Work out the finished part from the listing and answer in its coordinate system (mm). A direction names the side the tool comes from. Coordinates: 2 decimals unless noted, no trailing zeros. Write each loop counter-clockwise with the first axis right and the second up, starting at its lowest first coordinate (ties: lowest second). Pieces come first, ordered by that corner, then holes. Notation, with made-up numbers: M -7.5,50.25 L 36.5,50.25 A15 ccw 36.5,66.25 Z; hole C 1,4.5 d4. An arc over 180 degrees is marked long. Use CSV: the item, a comma, the result in double quotes.
from build123d import *

# Parameters (mm, degrees)
F0_W     = 8
F0_H     = 4
F1_DEPTH = 10
F2_R     = 2.6
F3_DEPTH = 21
F4_R     = 2.6
F5_DEPTH = 50
F6_R     = 3


with BuildPart() as f1:
    # F0 (on Top) → F1 (new body)
    with BuildSketch(Plane.XY):
        with BuildLine():
            Line((20.489401, 8.474669), (20.489401, 14.474669))
            Line((20.489401, 14.474669), (5.543822, 14.474669))
            Line((5.543822, 14.474669), (5.543822, 34.474669))
            Line((5.543822, 34.474669), (-1.356178, 34.474669))
            Line((-1.356178, 34.474669), (-1.356178, 22.474669))
            Line((-1.356178, 22.474669), (-8.556178, 22.474669))
            Line((-8.556178, 22.474669), (-8.556178, 34.474669))
            Line((-8.556178, 34.474669), (-15.456178, 34.474669))
            Line((-15.456178, 34.474669), (-15.456178, 1.16472))
            ThreePointArc((-15.456178, 1.16472), (-11.149904, -10.767062), (0.624203, -15.487426))
            Line((0.624203, -15.487426), (11.585323, -15.487426))
            Line((11.585323, -15.487426), (20.489401, -15.487426))
            Line((20.489401, -15.487426), (20.489401, -7.487426))
            Line((20.489401, -7.487426), (8.728599, -7.487426))
            ThreePointArc((8.728599, -7.487426), (-11.479476, -0.686755), (7.773673, 8.474669))
            Line((7.773673, 8.474669), (20.489401, 8.474669))
        make_face()
        with Locations((13.989401, -11.487426)):
            Rectangle(F0_W, F0_H, mode=Mode.SUBTRACT)
    extrude(amount=F1_DEPTH)

    # F2 (on face) → F3 (cut, through all)
    with BuildSketch(Plane.YZ.offset(5.543822)):
        with BuildLine():
            ThreePointArc((34.474669, 5), (33.010203, 1.464466), (29.474669, 0))
            Line((29.474669, 0), (34.474669, 0))
            Line((34.474669, 0), (34.474669, 5))
        make_face()
        with BuildLine():
            ThreePointArc((29.474669, 10), (33.010203, 8.535534), (34.474669, 5))
            Line((34.474669, 5), (34.474669, 10))
            Line((34.474669, 10), (29.474669, 10))
        make_face()
        with Locations((29.474669, 5)):
            Circle(F2_R)
    extrude(amount=-F3_DEPTH, mode=Mode.SUBTRACT)

    # F4 (on face) → F5 (cut, symmetric)
    with BuildSketch(Plane(origin=(0, -13.487426, 0), x_dir=(-1, 0, 0), z_dir=(0, 1, 0))):
        with Locations((-13.989401, 5)):
            Circle(F4_R)
    extrude(amount=F5_DEPTH, both=True, mode=Mode.SUBTRACT)

    # F6
    f6_edges = [f1.edges().sort_by_distance(p)[0] for p in [
        (20.489401, 14.474669, 5),
        (20.489401, -7.487426, 5),
        (20.489401, -15.487426, 5),
    ]]
    fillet(f6_edges, radius=F6_R)


solid = f1.part
Item 1: A tool of negligible diameter and unlimited length cuts with its end or side. For faces 1 (the face through (-5, 22.475, 5)), 2 (the face through (5.544, 24, 5)), 3 (the face through (17.989, -12, 5)), 4 (the face through (15.5, 8.475, 2.7)), from which of +Z, -Z, +X, -X, +Y, -Y can it reach the whole face along a straight path? Write none if from no direction.
Answer:
face 1,"+Z, -Z, +Y"
face 2,"+Z, -Z, +X, +Y"
face 3,"+Z, -Z"
face 4,"+Z, -Z, +X"
Item 2: Consider probe 1 along Y at (x, z) = (16, 0.75); probe 2 along X at (y, z) = (28.5, 2); probe 3 along X at (y, z) = (10.5, 4.75). Determine where each line is inside the solid, lowest interval first.
Answer:
probe 1,"y = -15.49 to -13.49, -9.49 to -7.49, 8.47 to 14.47"
probe 2,"x = -15.46 to -8.56, -1.36 to 5.54"
probe 3,"x = -15.46 to -4.69, 4.69 to 11.4, 16.58 to 20.49"
Item 3: For a pull along Y with two mould halves and no side action, classify faces 5 (the face through (10, 14.475, 5)), 6 (the face through (-15.456, 18, 5)), 7 (the face through (9.989, -12, 5)) as released by +Y, released by -Y, zero draft, split by the parting line, or undercut.
Answer:
face 5,"released by +Y"
face 6,"zero draft"
face 7,"undercut"
Item 4: Given pin 1 (5 mm diameter, centred on y = -6, z = 2, fed in from -X); pin 2 (1 mm diameter, centred on x = -9, z = 7.5, fed in from +Y); pin 3 (2.5 mm diameter, centred on x = 12, z = 2.5, fed in from +Y), each flat-ended and moving along its own axis, determine where each tip first touches the part or whether it passes through.
Answer:
pin 1,"stops at x = -15.1"
pin 2,"stops at y = 34.06"
pin 3,"stops at y = 14.47"
Item 5: The part is cut by section B-B (y = 24.5). Write down the section's boundary in (x, z).
Answer:
outline,"M -15.46,0 L -8.56,0 L -8.56,10 L -15.46,10 Z; M -1.36,0 L 5.54,0 L 5.54,10 L -1.36,10 Z"
Item 6: The part is cut by section C-C (x = 12). Write down the section's boundary in (y, z), then the cut area to 3 significant figures.
Answer:
outline,"M -15.49,0 L -13.49,0 L -13.49,3.33 L -15.49,3.33 Z; M -15.49,6.67 L -13.49,6.67 L -13.49,10 L -15.49,10 Z; M -9.49,0 L -7.49,0 L -7.49,3.33 L -9.49,3.33 Z; M -9.49,6.67 L -7.49,6.67 L -7.49,10 L -9.49,10 Z; M 8.47,0 L 14.47,0 L 14.47,3.33 L 8.47,3.33 Z; M 8.47,6.67 L 14.47,6.67 L 14.47,10 L 8.47,10 Z"
area,"66.5 mm2"
Item 7: The part is cut by section A-A (x = 0). Write down the section's boundary in (y, z), then the cut area to 3 significant figures.
Answer:
outline,"M -15.5,0 L -11.5,0 L -11.5,10 L -15.5,10 Z; M 11.5,0 L 29.47,0 A5 ccw 29.47,10 L 11.5,10 Z; hole C 29.47,5 d5.2"
area,"238 mm2"
Item 8: The part is cut by section D-D (x = -4.5). Write down the section's boundary in (y, z).
Answer:
outline,"M -14.83,0 L -10.58,0 L -10.58,10 L -14.83,10 Z; M 10.58,0 L 22.47,0 L 22.47,10 L 10.58,10 Z"
